Can you work these out from the model? Positions are in its coordinate system, mm. A direction names the side the tool comes from. Coordinates: 2 decimals unless noted, no trailing zeros. Order: outer loops, then holes, each group sorted by start corner. A loop starts at its lowest first (then second) coordinate and runs counter-clockwise, first axis right, second up.
```python
from build123d import *

# Parameters (mm, degrees)
F0_R     = 12.5
F1_DEPTH = 140
F3_DEPTH = 553
F4_R     = 12.5
F5_DEPTH = 487


with BuildPart() as f1:
    # F0 (on Top) → F1 (new body)
    with BuildSketch(Plane.XY):
        Circle(F0_R)
    extrude(amount=F1_DEPTH)

    # F2 (on face) → F3 (join)
    with BuildSketch(Plane.XY.offset(140)):
        Polygon((7.2168783649, 12.5), (-7.2168783649, 12.5), (-14.4337567297, 0), (-7.2168783649, -12.5), (7.2168783649, -12.5), (14.4337567297, 0), align=None)
    extrude(amount=F3_DEPTH)

    # F4 (on face) → F5 (join)
    with BuildSketch(Plane.XY.offset(693)):
        Circle(F4_R)
    extrude(amount=F5_DEPTH)


solid = f1.part
```
1. I'm going to push flat-ended pins straight in: pin 1 (1.8 mm diameter, centred on x = -13.5, y = -0.5, fed in from +Z); pin 2 (1 mm diameter, centred on y = 9, z = 651, fed in from +X); pin 3 (12 mm diameter, centred on y = 3.5, z = 534.5, fed in from +X). Where does each tip first touch, or does it pass through?
Completed:
pin 1: stops at z = 693
pin 2: stops at x = 9.53
pin 3: stops at x = 14.43
2. Imagine slicing it at A-A on z = 425. Please give me the cut outline in (x, y), then the cut area to 3 significant figures.
Completed:
outline: (-14.43, 0) - (-7.22, -12.5) - (7.22, -12.5) - (14.43, 0) - (7.22, 12.5) - (-7.22, 12.5) - close
area: 541 mm2
3. On a 3-axis mill with a long thin cutter (end or side, diameter ignored), from which of +Z, -Z, +X, -X, +Y, -Y can I reach the whole of each face in a straight line? I mean faces 1 (the flat face through (0, 0, 1180)), 2 (the cylindrical face through (11.923, 3.755, 69.02)), 3 (the cylindrical face through (11.923, 3.755, 933.091)). Say none if no direction works.
Completed:
face 1: +Z, +X, -X, +Y, -Y
face 2: -Z
face 3: +Z
4. Imagine slicing it at B-B on z = 991. Please give me the cut outline in (x, y), then the cut area to 3 significant figures.
Completed:
outline: circle Ø25 at (0, 0)
area: 491 mm2
5. Please list where these lines run through material, in increasing order: probe 1 along Z at (x, y) = (-13, 1); probe 2 along Y at (x, z) = (6.5, 78.5); probe 3 along Y at (x, z) = (-1, 845).
Completed:
probe 1: z = 140 to 693
probe 2: y = -10.68 to 10.68
probe 3: y = -12.46 to 12.46
